Geometry check sheet. Reference: drawing and pictorial views, mm from the part's lowest x, y, z. A direction names the side the tool comes from. Coordinates: 2 decimals unless noted, no trailing zeros. Loops run counter-clockwise (first coordinate to the right, second up) from the corner with the lowest first, then second, coordinate; pieces in that order, holes last. Notation, with made-up numbers: (15, 48) -> (58, 48) arc R13 ccw to (58, 61) -> close; hole circle Ø9 at (3.25, 14). An arc over 180 degrees is marked (long way). Use one line per item in the form item = value.
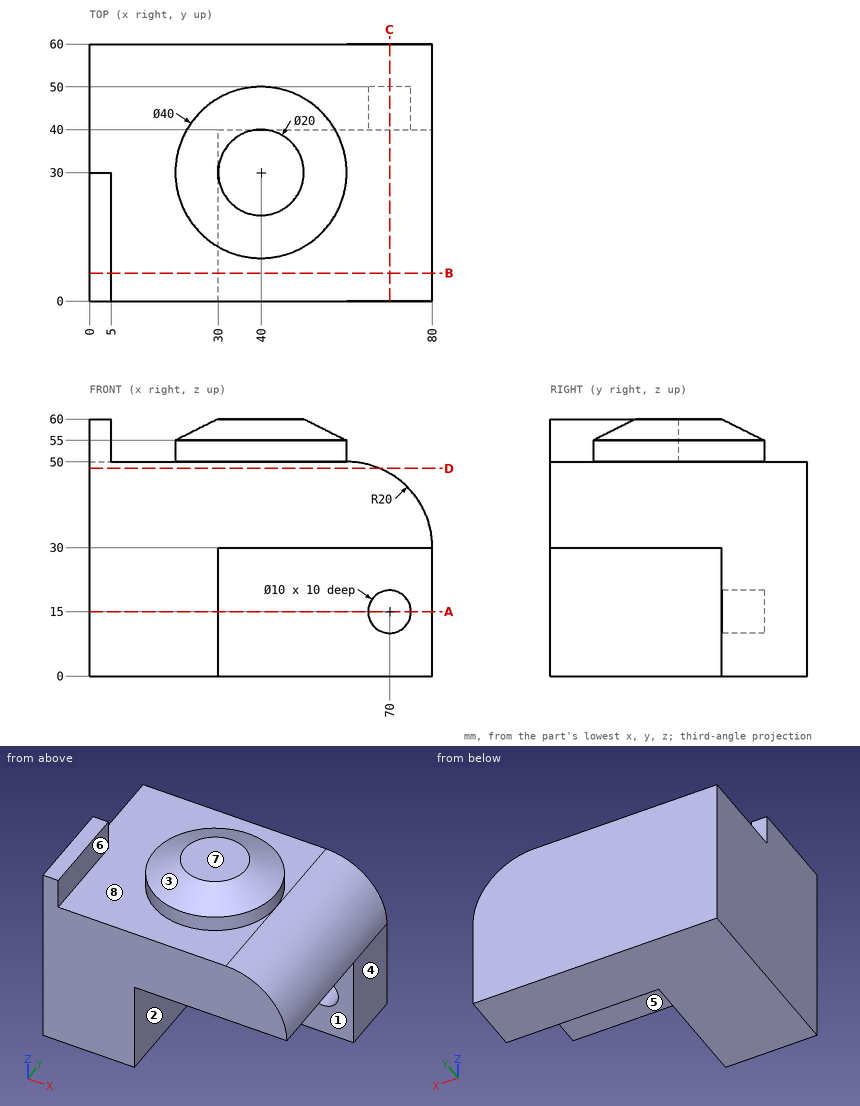
(1) Section check C-C, the plane x = 70. Record the boundary of the cut face in (y, z), plus the area to 3 significant figures.
Established:
outline = (0, 30) -> (40, 30) -> (40, 20) -> (50, 20) -> (50, 10) -> (40, 10) -> (40, 0) -> (60, 0) -> (60, 47.32) -> (0, 47.32) -> close
area = 1,540 mm²
(2) Mould release check, pull along X, two halves, no side actions. Record for the marked faces 1, 2 and 3: +X half, -X half, draft (parallel to the pull), parting line (faces both ways), or undercut.
Established:
face_1 = draft
face_2 = +X half
face_3 = undercut
(3) Section check A-A, the plane z = 15. Record the boundary of the cut face in (x, y).
Established:
outline = (0, 0) -> (30, 0) -> (30, 40) -> (65, 40) -> (65, 50) -> (75, 50) -> (75, 40) -> (80, 40) -> (80, 60) -> (0, 60) -> close
(4) Go/stop test with flat-tipped pins: P1, Ø12, axis at x = 47, y = 28.5, coming from the -Z side; P2, Ø5, axis at y = 18, z = 54, coming from the +X side; P3, Ø4, axis at x = 2.5, z = 55.5, coming from the +Y side. Record where each tip stops, or that it passes through.
Established:
P1 = 30
P2 = 57.6
P3 = 30
(5) Tool access check on the marked faces 4, 5, 6, 7 and 8. Record the directions out of +Z, -Z, +X, -X, +Y, -Y that give a thin tool (end or side, any length) a straight path to the whole face; none if there is none.
Established:
face_4 = +Z, -Z, +X, +Y, -Y
face_5 = -Z, +X, -Y
face_6 = +Z, +Y, -Y
face_7 = +Z, +X, -X, +Y, -Y
face_8 = +Z
(6) Scan lines: line 1 along Y through (x, z) = (54, 20); line 2 along Z through (x, y) = (29, 13); line 3 along X through (y, z) = (32, 21.5). Record each from-to range of solid material in increasing order.
Established:
line_1 = 40 to 60
line_2 = 0 to 50
line_3 = 0 to 30
(7) Section check B-B, the plane y = 6.5. Record the boundary of the cut face in (x, z).
Established:
outline = (0, 0) -> (30, 0) -> (30, 30) -> (80, 30) arc R20 ccw to (60, 50) -> (5, 50) -> (5, 60) -> (0, 60) -> close
(8) Section check D-D, the plane z = 48.5. Record the boundary of the cut face in (x, y), plus the area to 3 significant figures.
Established:
outline = (0, 0) -> (67.6, 0) -> (67.6, 60) -> (0, 60) -> close
area = 4,060 mm²
